Autodesk Inventor part; units mm, degrees
ref_plane "YZ Plane" through (0, 0, 0) normal (1, 0, 0) x (0, 1, 0)
ref_plane "XZ Plane" through (0, 0, 0) normal (0, 1, 0) x (-1, 0, 0)
ref_plane "XY Plane" through (0, 0, 0) normal (0, 0, 1) x (1, 0, 0)
sketch "Sketch1" plane through (0, 0, 0) normal (0, 0, 1) x (1, 0, 0)
  line L0 (12.7, 25.019) -> (-12.7, 25.019)
  line L1 (-12.7, 25.019) -> (-12.7, -25.019)
  line L2 (-12.7, -25.019) -> (12.7, -25.019)
  line L3 (12.7, -25.019) -> (12.7, 25.019)
  point P0 (0, 0)
  point P1 (-12.7, 0)
  point P2 (0, 25.019)
  dimension "d0" = 25.4
  dimension "d1" = 50.038
extrude "Extrusion1" add sketch "Sketch1" along normal blind 8.382
sketch "Sketch2" plane through (-12.7, 25.019, 0) normal (0, 1, 0) x (1, 0, 0)
  line L0 (0, 0) -> (0, -8.382)
  circle A0 centre (9.144, -4.191) radius 3.4611
  point P0 (12.7, 0)
  dimension "d4" = 9.144
extrude "Extrusion2" add sketch "Sketch2" along normal blind 11.43
properties part number "Video Tx"
Could you check a few things on this model? Use its own coordinates, in mm. A direction names the side the tool comes from. Give positions to 0.01 mm unless a question says otherwise; leave off trailing zeros. Order: outer loops, then holes, each group sorted by start corner. A loop starts at its lowest first (then second) coordinate and runs counter-clockwise, first axis right, second up. Notation, with made-up numbers: (-23.75, -6.75) - (3.25, -6.75) arc R28 cw to (3.25, 11.25) - close; hole circle Ø3 at (15, -34). An arc over 180 degrees is marked (long way). Return JSON: item names as keys, results as strings. Group by question number.
Q1. Suppose I cut it at A-A, the plane z = 6.5. Please give me the cut outline in (x, y).
Q2. Suppose I cut it at C-C, the plane x = -9.5. Please give me the cut outline in (y, z).
Q3. Suppose I cut it at B-B, the plane x = -1.75. Please give me the cut outline in (y, z), and give its area (3 significant figures).
Q4. Please list where these lines run through material, in increasing order: line 1 along Y through (x, z) = (6.25, 6.75); line 2 along X through (y, z) = (26.5, 1.5). Write a range as [from, to].
Q5. Which directions (+Z, -Z, +X, -X, +Y, -Y) give clear straight access to the entire face, cutting with the end or side of a thin tool? Please do faces 1 (the face through (-1.695, 30.654, 7.109)), 2 (the face through (0, -25.019, 4)).
Resolved:
{
 "1": {"outline": "(-12.7, -25.02) - (12.7, -25.02) - (12.7, 25.02) - (-0.98, 25.02) - (-0.98, 36.45) - (-6.13, 36.45) - (-6.13, 25.02) - (-12.7, 25.02) - close"},
 "2": {"outline": "(-25.02, 0) - (25.02, 0) - (25.02, 8.38) - (-25.02, 8.38) - close"},
 "3": {"outline": "(-25.02, 0) - (25.02, 0) - (25.02, 1.24) - (36.45, 1.24) - (36.45, 7.14) - (25.02, 7.14) - (25.02, 8.38) - (-25.02, 8.38) - close", "area": "487 mm2"},
 "4": {"line 1": "y = [-25.02, 25.02]", "line 2": "x = [-5.73, -1.38]"},
 "5": {"face 1": "+Y", "face 2": "+Z, -Z, +X, -X, -Y"}
}
